from build123d import *

# Parameters (mm, degrees)
SKETCH1_W           = 44.45
SKETCH1_H           = 12.7
SKETCH1_W_2         = 12.7
BOSS_EXTRUDE1_DEPTH = 12.7
SKETCH2_R           = 3.175
CUT_EXTRUDE1_DEPTH  = 25.4
SKETCH3_R           = 3.175
CUT_EXTRUDE2_DEPTH  = 25.4
SKETCH4_W           = 12.7
SKETCH4_H           = 12.7
BOSS_EXTRUDE2_DEPTH = 15.875
BOSS_EXTRUDE3_START = 12.7
SKETCH5_W           = 44.45
SKETCH5_H           = 12.7
SKETCH5_R           = 3.175
BOSS_EXTRUDE3_DEPTH = 12.7
SKETCH6_W           = 44.45
SKETCH6_H           = 12.7
CUT_EXTRUDE3_DEPTH  = 12.7
CUT_EXTRUDE4_REACH  = 57.54
SKETCH7_R           = 3.175


with BuildPart() as part:
    # Sketch1 → Boss-Extrude1 (new body)
    with BuildSketch(Plane.XY):
        with Locations((0, -6.35)):
            Rectangle(SKETCH1_W, SKETCH1_H)
        with Locations((0, 6.35)):
            Rectangle(SKETCH1_W, SKETCH1_H)
        with Locations((-28.575, 6.35)):
            Rectangle(SKETCH1_W_2, SKETCH1_H)
        with Locations((28.575, 6.35)):
            Rectangle(SKETCH1_W_2, SKETCH1_H)
    extrude(amount=BOSS_EXTRUDE1_DEPTH)

    # Sketch2 → Cut-Extrude1 (cut)
    with BuildSketch(Plane.XZ.offset(12.7)):
        with Locations(Location((-15.875, 6.35, 0), (0, 0, 270))):
            Circle(SKETCH2_R)
        with Locations(Location((15.875, 6.35, 0), (0, 0, 270))):
            Circle(SKETCH2_R)
    extrude(amount=-CUT_EXTRUDE1_DEPTH, mode=Mode.SUBTRACT)

    # Sketch3 → Cut-Extrude2 (cut)
    with BuildSketch(Plane.XZ):
        with Locations(Location((-28.575, 6.35, 0), (0, 0, 270))):
            Circle(SKETCH3_R)
        with Locations(Location((28.575, 6.35, 0), (0, 0, 270))):
            Circle(SKETCH3_R)
    extrude(amount=-CUT_EXTRUDE2_DEPTH, mode=Mode.SUBTRACT)

    # Sketch4 → Boss-Extrude2 (add)
    with BuildSketch(Plane.XZ.offset(12.7)):
        with Locations((0, 6.35)):
            Rectangle(SKETCH4_W, SKETCH4_H)
    extrude(amount=BOSS_EXTRUDE2_DEPTH)

    # Sketch5 → Boss-Extrude3 (add)
    with BuildSketch(Plane.XZ.offset(28.575).offset(BOSS_EXTRUDE3_START)):
        with Locations((0, 6.35)):
            Rectangle(SKETCH5_W, SKETCH5_H)
        with Locations(Location((-15.875, 6.35, 0), (0, 0, 270))):
            Circle(SKETCH5_R, mode=Mode.SUBTRACT)
        with Locations(Location((15.875, 6.35, 0), (0, 0, 270))):
            Circle(SKETCH5_R, mode=Mode.SUBTRACT)
    extrude(amount=-BOSS_EXTRUDE3_DEPTH)

    # Sketch6 → Cut-Extrude3 (cut)
    with BuildSketch(Plane.XZ.offset(41.275)):
        with Locations((0, 6.35)):
            Rectangle(SKETCH6_W, SKETCH6_H)
    extrude(amount=-CUT_EXTRUDE3_DEPTH, mode=Mode.SUBTRACT)

    # Sketch7 → Cut-Extrude4 (cut, up to next)
    with BuildSketch(Plane.XZ.offset(28.575), mode=Mode.PRIVATE) as cut_extrude4_sk1:
        with Locations(Location((0, 6.35, 0), (0, 0, 270))):
            Circle(SKETCH7_R)
    cut_extrude4_tool1 = extrude(cut_extrude4_sk1.sketch, amount=-CUT_EXTRUDE4_REACH, mode=Mode.PRIVATE) & part.part
    add(cut_extrude4_tool1.solids().sort_by_distance((0, -28.575, 6.35))[0], mode=Mode.SUBTRACT)


solid = part.part
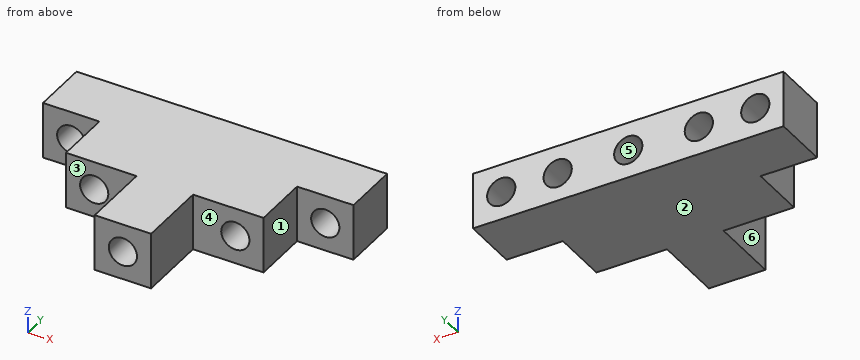
Part model, mm, in its own coordinate system. Face numbers are marked on the shaded views. A direction names the side the tool comes from. Give positions to 0.01 mm unless a question says otherwise; leave off trailing zeros. Order: outer loops, then holes, each group sorted by start corner. A loop starts at its lowest first (then second) coordinate and runs counter-clockwise, first axis right, second up. Notation, with made-up numbers: (-6.5, 53.25) - (33.5, 53.25) arc R32 cw to (33.5, 81.25) - close; hole circle Ø9 at (8, -31.5). An arc over 180 degrees is marked (long way). Use a Markdown table: item, result.
1) Saw through at B-B on x = 0. List the corners of the cut face in (y, z) (3 decimals), plus the area to 3 significant figures.
Checked values:
| item | result |
|---|---|
| outline | (-28.575, 0) - (12.7, 0) - (12.7, 3.175) - (-28.575, 3.175) - close; (-28.575, 9.525) - (12.7, 9.525) - (12.7, 12.7) - (-28.575, 12.7) - close |
| area | 262 mm² |
2) Saw through at D-D on z = 1.25. List the corners of the cut face in (x, y) (3 decimals), plus the area to 3 significant figures.
Checked values:
| item | result |
|---|---|
| outline | (-34.925, 0) - (-22.225, 0) - (-22.225, -12.7) - (-6.35, -12.7) - (-6.35, -28.575) - (6.35, -28.575) - (6.35, -12.7) - (22.225, -12.7) - (22.225, 0) - (34.925, 0) - (34.925, 12.7) - (-34.925, 12.7) - close |
| area | 1,650 mm² |
3) Two-plate mould, pull along X, no slides. Class the marked faces 4, 5 and 6: +X half, -X half, draft (parallel to the pull), parting line (faces both ways), or undercut.
Checked values:
| item | result |
|---|---|
| face 4 | draft |
| face 5 | undercut |
| face 6 | -X half |
4) 3-axis set-ups, long thin cutter, end or side, ignore diameter. For the marked faces 1, 2 and 3: which of +Z, -Z, +X, -X, +Y, -Y reach the whole face in a straight line?
Checked values:
| item | result |
|---|---|
| face 1 | +Z, -Z, +X, -Y |
| face 2 | -Z, +X, -X, +Y, -Y |
| face 3 | +Z, -Z, -X, -Y |
5) Probe L1, parallel to X at y = 3.25, z = 6.35 (3 decimals); L2, parallel to X at y = -5, z = 6.35 (3 decimals); L3, parallel to X at y = 5.5, z = 4 (3 decimals). List the from-to ranges inside material, lowest first. Write a range as from..to.
Checked values:
| item | result |
|---|---|
| L1 | -34.925..-31.75, -25.4..-19.05, -12.7..-3.175, 3.175..12.7, 19.05..25.4, 31.75..34.925 |
| L2 | -22.225..-19.05, -12.7..-3.175, 3.175..12.7, 19.05..22.225 |
| L3 | -34.925..-30.71, -26.44..-18.01, -13.74..-2.135, 2.135..13.74, 18.01..26.44, 30.71..34.925 |
6) Saw through at A-A on z = 6.35. Count the separate pieces of the cut face and the enclosed holes in it, plus the area to 3 significant figures.
Checked values:
| item | result |
|---|---|
| separate pieces | 6 |
| enclosed holes | 0 |
| area | 907 mm² |
7) Saw through at C-C on y = -2. List the corners of the cut face in (x, z) (3 decimals), plus the area to 3 significant figures.
Checked values:
| item | result |
|---|---|
| outline | (-22.225, 0) - (22.225, 0) - (22.225, 12.7) - (-22.225, 12.7) - close; hole circle Ø6.35 at (-15.875, 6.35); hole circle Ø6.35 at (0, 6.35); hole circle Ø6.35 at (15.875, 6.35) |
| area | 470 mm² |
8) Flat gauge pins, fed straight in: P1, Ø4, axis at x = 14, z = 9, coming from the -Y side; P2, Ø5, axis at x = -7.5, z = 4, coming from the -Y side (3 decimals); P3, Ø6.5, axis at y = -22.5, z = 4.5, coming from the +X side; P4, Ø4, axis at x = 28, z = 3.5, coming from the -Y side. Where does each tip first touch, or does it go through?
Checked values:
| item | result |
|---|---|
| P1 | y = -12.7 |
| P2 | y = -28.575 |
| P3 | x = 6.35 |
| P4 | y = 0 |
